The listing builds one solid part. Answer for the finished solid, in the listing's coordinates (mm). Face numbers are marked on the shaded views. A direction names the side the tool comes from. Round coordinates to 2 decimals unless told otherwise and drop trailing zeros. Loops run counter-clockwise (first coordinate to the right, second up) from the corner with the lowest first, then second, coordinate; pieces in that order, holes last. Notation, with made-up numbers: (71.5, -7) - (84.5, -7) arc R23 cw to (84.5, 7) - close; hole circle Ø10 at (49, 56.25). An arc over 180 degrees is marked (long way). Write item = value, one per line. Start each with the question number.
1) Section C-C, the plane z = 7.75 is taken. Determine the outline of the cut face in (x, y).
2) A tool of negligible diameter and unlimited length cuts with its end or side. For the marked faces 1, 2, 3, 4 and 5, from which of +Z, -Z, +X, -X, +Y, -Y can it reach the whole face along a straight path? Write none if from no direction.
3) Given pin 1 Ø1.8 at (x, y) = (8, 3) entering from +Z; pin 2 Ø1.5 at (y, z) = (5.5, 8.5) entering from -X; pin 3 Ø2.5 at (y, z) = (2.5, -8) entering from +X; pin 4 Ø3 at (x, z) = (-10.065, 0) entering from +Y, each flat-ended and moving along its own axis, determine where each tip first touches the part or whether it passes through.
4) Section B-B, the plane y = 2.85 is taken. Determine the outline of the cut face in (x, z) (3 decimals), and give its area (3 significant figures).
5) Section A-A, the plane z = 0 is taken. Determine the outline of the cut face in (x, y) (3 decimals), and give its area (3 significant figures).
6) Straight lines are drawn through the part: line 1 along X through (y, z) = (2.7, 0.25); line 2 along X through (y, z) = (2.45, -1.25); line 3 along Z through (x, y) = (-8, 0.3). For each, find the intervals that lie inside material, in ascending order.
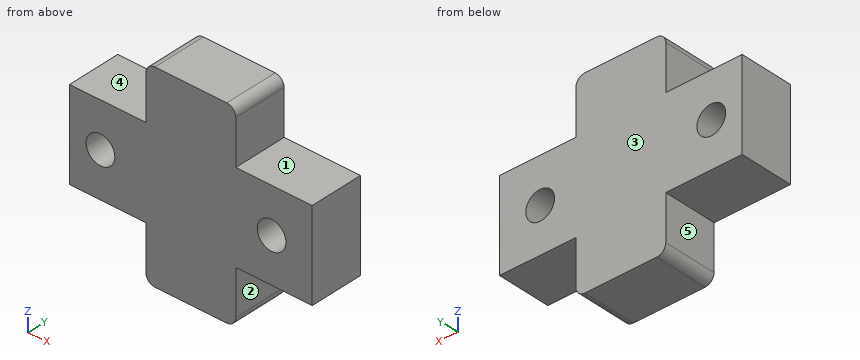
from build123d import *

# Parameters (mm, degrees)
SKETCH1_W              = 27
SKETCH1_H              = 10
BOSS_EXTRUDE1_DEPTH    = 6
M3_CLEARANCE_HOLE1_D   = 3.2
SKETCH234_W            = 10
SKETCH234_H            = 6
BOSS_EXTRUDE234_DEPTH  = 6
FILLET134_R            = 1
FILLET134_OF_MIRROR1_R = 1


with BuildPart() as part:
    # Sketch1 → Boss-Extrude1 (new body)
    with BuildSketch(Plane(origin=(0, 0, 0), x_dir=(1, 0, 0), z_dir=(0, 1, 0))):
        Rectangle(SKETCH1_W, SKETCH1_H)
    extrude(amount=BOSS_EXTRUDE1_DEPTH)

    # M3 Clearance Hole1 (through all)
    with Locations(Plane(origin=(0, 0, 0), x_dir=(-1, 0, 0), z_dir=(0, -1, 0))):
        with Locations((10.065, 0), (-8.985, 0)):
            Hole(M3_CLEARANCE_HOLE1_D / 2)

    # Sketch234 → Boss-Extrude234 (add)
    with BuildSketch(Plane(origin=(0.767778608, 6, 5), x_dir=(-1, 0, 0), z_dir=(0, 0, 1))):
        with Locations((0.767778608, 3)):
            Rectangle(SKETCH234_W, SKETCH234_H)
    boss_extrude234 = extrude(amount=BOSS_EXTRUDE234_DEPTH)

    # Fillet134
    fillet134_edges = [part.edges().sort_by_distance(p)[0] for p in [
        (5, 3, 11),
        (-5, 3, 11),
    ]]
    fillet(fillet134_edges, radius=FILLET134_R)

    # Mirror1: Boss-Extrude234 across plane
    add(boss_extrude234.mirror(Plane.XY))

    # Fillet134 of Mirror1
    fillet134_of_mirror1_edges = [part.edges().sort_by_distance(p)[0] for p in [
        (5, 3, -11),
        (-5, 3, -11),
    ]]
    fillet(fillet134_of_mirror1_edges, radius=FILLET134_OF_MIRROR1_R)


solid = part.part
Geometry check:
q1.outline = (-5, 0) - (5, 0) - (5, 6) - (-5, 6) - close
q2.face_1 = +Z, +X, +Y, -Y
q2.face_2 = -Z, +X, +Y, -Y
q2.face_3 = +Z, -Z, +X, -X, +Y
q2.face_4 = +Z, -X, +Y, -Y
q2.face_5 = -Z, -X, +Y, -Y
q3.pin_1 = 5
q3.pin_2 = -5
q3.pin_3 = 5
q3.pin_4 = through
q4.outline = (-13.5, -5) - (-5, -5) - (-5, -10) arc R1 ccw to (-4, -11) - (4, -11) arc R1 ccw to (5, -10) - (5, -5) - (13.5, -5) - (13.5, 5) - (5, 5) - (5, 10) arc R1 ccw to (4, 11) - (-4, 11) arc R1 ccw to (-5, 10) - (-5, 5) - (-13.5, 5) - close; hole circle Ø3.2 at (-10.065, 0); hole circle Ø3.2 at (8.985, 0)
q4.area = 373 mm2
q5.outline = (-13.5, 0) - (-11.665, 0) - (-11.665, 6) - (-13.5, 6) - close; (-8.465, 0) - (7.385, 0) - (7.385, 6) - (-8.465, 6) - close; (10.585, 0) - (13.5, 0) - (13.5, 6) - (10.585, 6) - close
q5.area = 124 mm2
q6.line_1 = -13.5 to -11.65, -8.48 to 7.4, 10.57 to 13.5
q6.line_2 = -13.5 to -11.06, -9.07 to 7.99, 9.98 to 13.5
q6.line_3 = -5 to 5
